For this review, take the finished solid that the model builds, in its own axes (mm). A direction names the side the tool comes from. Coordinates: 2 decimals unless noted, no trailing zeros. Loops run counter-clockwise (first coordinate to the right, second up) from the corner with the lowest first, then second, coordinate; pieces in that order, holes last. Notation, with made-up numbers: M 15.25,84.25 L 57.25,84.25 A30 ccw 57.25,109.25 Z; hole C 6.25,75 d10. An arc over 180 degrees is marked long. Answer as a JSON object with one key per item and string values. Group by question number.
Item 1: Add section A-A (z = 17.5). State the section outline as (x, y) points.
Item 2: Add section C-C (z = 11.5). State the section outline as (x, y) points, then the cut area to 3 significant figures.
Item 3: Wall thickness on L1, parallel to Z at x = 18, y = 5.5; L2, parallel to X at y = 14.5, z = 22; L3, parallel to Z at x = -40, y = -8.5: over which ranges is each line inside the solid? List them lowest first. Write a range as from..to.
Item 4: Insertion check: pin 1 (16 mm diameter, centred on x = -41, z = 13, fed in from +Y); pin 2 (20 mm diameter, centred on y = 9.5, z = 25, fed in from +X); pin 3 (12 mm diameter, centred on x = 0.5, y = 6.5, fed in from +Z); pin 4 (8 mm diameter, centred on x = -15.5, y = 1.5, fed in from -Z). Each pin has a flat end and moves straight along its axis. Give the tip position at first contact, or say it passes through.
Item 5: Mouldability with a two-part tool opening along Z and no side actions: class faces 1 (the face through (20, 0, 15)), 2 (the face through (27, -5, 35)), 3 (the face through (-44, -5, 13)) as +Z half, -Z half, draft (parallel to the pull), parting line (faces both ways), or undercut.
Item 6: Add section D-D (y = -11). State the section outline as (x, z) points.
Item 7: Tool access review of faces 4 (the face through (-20, 0, 15)), 5 (the face through (30, 7, 18)), 6 (the face through (-14, 19.974, 26)), 7 (the face through (-30, 7, 18)), 8 (the face through (12.5, 0, 30)): name each direction out of +Z, -Z, +X, -X, +Y, -Y from which nothing blocks a thin tool from reaching the whole face with its end or side.
Item 8: Add section B-B (x = -40). State the section outline as (y, z) points.
from build123d import *

# Parameters (mm, degrees)
ESBO_O1_W                = 60
ESBO_O1_H                = 40
RESSALTO_EXTRUS_O1_DEPTH = 35
ESBO_O3_W                = 40
ESBO_O3_H                = 20
CORTE_EXTRUS_O2_DEPTH    = 80
ESBO_O4_W                = 25
ESBO_O4_H                = 10
CORTE_EXTRUS_O3_DEPTH    = 80
ESBO_O5_W                = 35
ESBO_O5_H                = 15
RESSALTO_EXTRUS_O2_DEPTH = 20
ESBO_O6_W                = 35
ESBO_O6_H                = 15
RESSALTO_EXTRUS_O3_DEPTH = 20
ESBO_O7_W                = 60
ESBO_O7_H                = 35
RESSALTO_EXTRUS_O4_DEPTH = 10
ESBO_O8_R                = 5
CORTE_EXTRUS_O4_DEPTH    = 51
ESBO_O9_W                = 60
ESBO_O9_H                = 10.026146623
CORTE_EXTRUS_O5_DEPTH    = 36


with BuildPart() as part:
    # Esboço1 → Ressalto-extrusão1 (new body)
    with BuildSketch(Plane.XY):
        Rectangle(ESBO_O1_W, ESBO_O1_H)
    extrude(amount=RESSALTO_EXTRUS_O1_DEPTH)

    # Esboço3 → Corte-extrusão2 (cut)
    with BuildSketch(Plane(origin=(0, 20, 0), x_dir=(1, 0, 0), z_dir=(0, 1, 0))):
        with Locations((0, -15)):
            Rectangle(ESBO_O3_W, ESBO_O3_H)
    extrude(amount=-CORTE_EXTRUS_O2_DEPTH, mode=Mode.SUBTRACT)

    # Esboço4 → Corte-extrusão3 (cut)
    with BuildSketch(Plane(origin=(0, 20, 0), x_dir=(1, 0, 0), z_dir=(0, 1, 0))):
        with Locations((0, -30)):
            Rectangle(ESBO_O4_W, ESBO_O4_H)
    extrude(amount=-CORTE_EXTRUS_O3_DEPTH, mode=Mode.SUBTRACT)

    # Esboço5 → Ressalto-extrusão2 (add)
    with BuildSketch(Plane(origin=(30, 0, 0), x_dir=(0, 0, -1), z_dir=(1, 0, 0))):
        with Locations((-17.5, -12.5)):
            Rectangle(ESBO_O5_W, ESBO_O5_H)
    extrude(amount=RESSALTO_EXTRUS_O2_DEPTH)

    # Esboço6 → Ressalto-extrusão3 (add)
    with BuildSketch(Plane.ZY.offset(30)):
        with Locations((17.5, -12.5)):
            Rectangle(ESBO_O6_W, ESBO_O6_H)
    extrude(amount=RESSALTO_EXTRUS_O3_DEPTH)

    # Esboço7 → Ressalto-extrusão4 (add)
    with BuildSketch(Plane(origin=(0, 20, 0), x_dir=(1, 0, 0), z_dir=(0, 1, 0))):
        with Locations((0, -17.5)):
            Rectangle(ESBO_O7_W, ESBO_O7_H)
    extrude(amount=RESSALTO_EXTRUS_O4_DEPTH)

    # Esboço8 → Corte-extrusão4 (cut, through all)
    with BuildSketch(Plane.XZ.offset(20)):
        with Locations((40, 17.5)):
            Circle(ESBO_O8_R)
        with Locations((-40, 17.5)):
            Circle(ESBO_O8_R)
    extrude(amount=-CORTE_EXTRUS_O4_DEPTH, mode=Mode.SUBTRACT)

    # Esboço9 → Corte-extrusão5 (cut, through all)
    with BuildSketch(Plane.XY.offset(35)):
        with Locations((0, 24.986926689)):
            Rectangle(ESBO_O9_W, ESBO_O9_H)
    extrude(amount=-CORTE_EXTRUS_O5_DEPTH, mode=Mode.SUBTRACT)


solid = part.part
From the geometry:
{
 "1": {"outline": "M -50,-20 L -45,-20 L -45,-5 L -50,-5 Z; M -35,-20 L -20,-20 L -20,19.97 L -30,19.97 L -30,-5 L -35,-5 Z; M 20,-20 L 35,-20 L 35,-5 L 30,-5 L 30,19.97 L 20,19.97 Z; M 45,-20 L 50,-20 L 50,-5 L 45,-5 Z"},
 "2": {"outline": "M -50,-20 L -20,-20 L -20,19.97 L -30,19.97 L -30,-5 L -50,-5 Z; M 20,-20 L 50,-20 L 50,-5 L 30,-5 L 30,19.97 L 20,19.97 Z", "area": "1,400 mm²"},
 "3": {"L1": "z = 0..5, 25..35", "L2": "x = -30..-20, 20..30", "L3": "z = 0..12.5, 22.5..35"},
 "4": {"pin 1": "stops at y = -5", "pin 2": "stops at x = 30", "pin 3": "stops at z = 5", "pin 4": "stops at z = 0"},
 "5": {"face 1": "undercut", "face 2": "+Z half", "face 3": "draft"},
 "6": {"outline": "M -50,0 L 50,0 L 50,35 L 12.5,35 L 12.5,25 L 20,25 L 20,5 L -20,5 L -20,25 L -12.5,25 L -12.5,35 L -50,35 Z; hole C -40,17.5 d10; hole C 40,17.5 d10"},
 "7": {"face 4": "+Y, -Y", "face 5": "+Z, -Z, +X, +Y", "face 6": "+Z, -Z, +X, -X, +Y", "face 7": "+Z, -Z, -X, +Y", "face 8": "+Z, +Y, -Y"},
 "8": {"outline": "M -20,0 L -5,0 L -5,12.5 L -20,12.5 Z; M -20,22.5 L -5,22.5 L -5,35 L -20,35 Z"}
}
